Print and shaded views of the part. All mm, measured from the part's lowest x, y and z. Round coordinates to 2 decimals unless told otherwise and drop trailing zeros. Loops run counter-clockwise (first coordinate to the right, second up) from the corner with the lowest first, then second, coordinate; pieces in that order, holes last. Notation, with made-up numbers: (6.5, -15.5) - (27.5, -15.5) arc R14 cw to (27.5, -5.5) - close; hole circle Ø10 at (6, 36.25). An arc over 180 degrees is marked (long way). Answer as a JSON object with one key per item and string values.
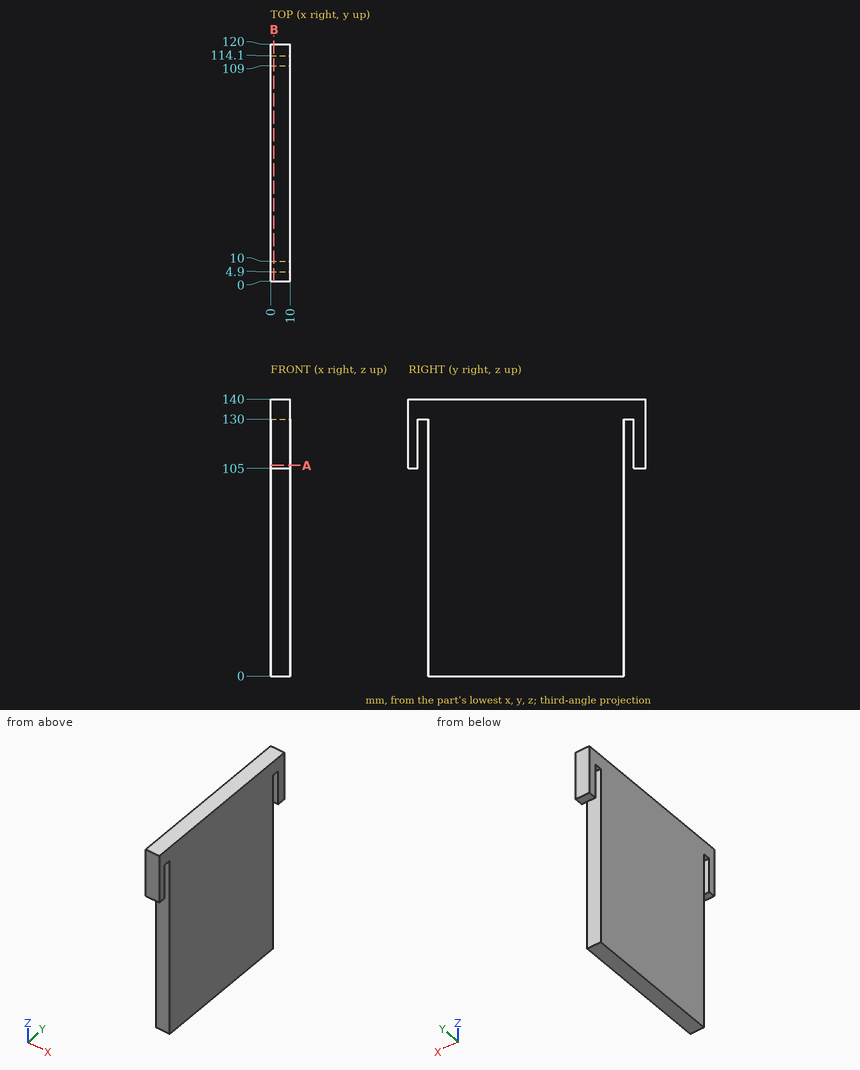
1) Probe probe 1 along Y at (x, z) = (4.75, 126.5); probe 2 along Y at (x, z) = (2, 36.5). List the from-to ranges inside material, lowest first.
Values follow:
{"probe 1": "0 to 4.9, 10 to 109, 114.1 to 120", "probe 2": "10 to 109"}
2) Slice it at B-B on x = 1.75. List the corners of the cut face in (y, z).
Values follow:
{"outline": "(0, 105) - (4.9, 105) - (4.9, 130) - (10, 130) - (10, 0) - (109, 0) - (109, 130) - (114.1, 130) - (114.1, 105) - (120, 105) - (120, 140) - (0, 140) - close"}
3) Slice it at A-A on z = 106.5. List the corners of the cut face in (x, y).
Values follow:
{"outline": "(0, 0) - (10, 0) - (10, 4.9) - (0, 4.9) - close; (0, 10) - (10, 10) - (10, 109) - (0, 109) - close; (0, 114.1) - (10, 114.1) - (10, 120) - (0, 120) - close"}
4) Drop flat-ended pins along their axis: P1, Ø2, axis at x = 2, y = 27.5, coming from the -Z side; P2, Ø2.5, axis at x = 6.5, y = 7.5, coming from the -Z side; P3, Ø4, axis at x = 2, z = 84, coming from the -Y side; P4, Ø1.5, axis at x = 5, y = 1, coming from the -Z side. Give the stop position or say it passes through.
Values follow:
{"P1": "z = 0", "P2": "z = 130", "P3": "y = 10", "P4": "z = 105"}
